```python
from build123d import *

# Parameters (mm, degrees)
CROQUIS1_W               = 28.88
CROQUIS1_H               = 55.3
CROQUIS1_R               = 1.5
SALIENTE_EXTRUIR8_DEPTH  = 3
CROQUIS19_W              = 28.88
CROQUIS19_H              = 55.3
CORTAR_EXTRUIR3_DEPTH    = 0.5
CROQUIS20_W              = 3
CROQUIS20_H              = 7.5
SALIENTE_EXTRUIR18_DEPTH = 23.5
SALIENTE_EXTRUIR19_START = -2.5
CROQUIS21_W              = 28.88
CROQUIS21_H              = 55.3
CROQUIS21_R              = 1.5
SALIENTE_EXTRUIR19_DEPTH = 2.5
CROQUIS22_R              = 1.5
CORTAR_EXTRUIR4_DEPTH    = 3
CROQUIS23_W              = 55.3
CROQUIS23_H              = 2.5
CORTAR_EXTRUIR5_DEPTH    = 68.588049239
CROQUIS24_W              = 55.3
CROQUIS24_H              = 23.5
SALIENTE_EXTRUIR20_DEPTH = 3


with BuildPart() as part:
    # Croquis1 → Saliente-Extruir8 (new body)
    with BuildSketch(Plane(origin=(0, 0, 0), x_dir=(1, 0, 0), z_dir=(0, 1, 0))):
        with Locations((14.44, 27.65)):
            Rectangle(CROQUIS1_W, CROQUIS1_H)
        with Locations(Location((14.44, 17.75, 0), (0, 0, 270))):
            Circle(CROQUIS1_R, mode=Mode.SUBTRACT)
        with Locations(Location((21.44, 17.75, 0), (0, 0, 270))):
            Circle(CROQUIS1_R, mode=Mode.SUBTRACT)
        with Locations(Location((14.44, 24.75, 0), (0, 0, 270))):
            Circle(CROQUIS1_R, mode=Mode.SUBTRACT)
        with Locations(Location((7.44, 17.75, 0), (0, 0, 270))):
            Circle(CROQUIS1_R, mode=Mode.SUBTRACT)
        with Locations(Location((14.44, 10.75, 0), (0, 0, 270))):
            Circle(CROQUIS1_R, mode=Mode.SUBTRACT)
        with Locations(Location((21.44, 37.55, 0), (0, 0, 90))):
            Circle(CROQUIS1_R, mode=Mode.SUBTRACT)
        with Locations(Location((14.44, 44.55, 0), (0, 0, 90))):
            Circle(CROQUIS1_R, mode=Mode.SUBTRACT)
        with Locations(Location((14.44, 30.55, 0), (0, 0, 90))):
            Circle(CROQUIS1_R, mode=Mode.SUBTRACT)
        with Locations(Location((14.44, 37.55, 0), (0, 0, 90))):
            Circle(CROQUIS1_R, mode=Mode.SUBTRACT)
        with Locations(Location((7.44, 37.55, 0), (0, 0, 90))):
            Circle(CROQUIS1_R, mode=Mode.SUBTRACT)
    extrude(amount=SALIENTE_EXTRUIR8_DEPTH)

    # Croquis19 → Cortar-Extruir3 (cut)
    with BuildSketch(Plane(origin=(0, 3, 0), x_dir=(1, 0, 0), z_dir=(0, 1, 0))):
        with Locations((14.44, 27.65)):
            Rectangle(CROQUIS19_W, CROQUIS19_H)
    extrude(amount=-CORTAR_EXTRUIR3_DEPTH, mode=Mode.SUBTRACT)

    # Croquis20 → Saliente-Extruir18 (add)
    with BuildSketch(Plane(origin=(0, 2.5, 0), x_dir=(1, 0, 0), z_dir=(0, 1, 0))):
        with Locations((1.5, 51.55)):
            Rectangle(CROQUIS20_W, CROQUIS20_H)
        with Locations((1.5, 3.75)):
            Rectangle(CROQUIS20_W, CROQUIS20_H)
    extrude(amount=SALIENTE_EXTRUIR18_DEPTH)

    # Croquis21 → Saliente-Extruir19 (add)
    with BuildSketch(Plane(origin=(0, 26, 0), x_dir=(1, 0, 0), z_dir=(0, 1, 0)).offset(SALIENTE_EXTRUIR19_START)):
        with Locations((14.44, 27.65)):
            Rectangle(CROQUIS21_W, CROQUIS21_H)
        with Locations(Location((14.44, 44.55, 0), (0, 0, 90))):
            Circle(CROQUIS21_R, mode=Mode.SUBTRACT)
        with Locations(Location((21.44, 37.55, 0), (0, 0, 90))):
            Circle(CROQUIS21_R, mode=Mode.SUBTRACT)
        with Locations(Location((14.44, 37.55, 0), (0, 0, 90))):
            Circle(CROQUIS21_R, mode=Mode.SUBTRACT)
        with Locations(Location((14.44, 30.55, 0), (0, 0, 90))):
            Circle(CROQUIS21_R, mode=Mode.SUBTRACT)
        with Locations(Location((7.44, 37.55, 0), (0, 0, 90))):
            Circle(CROQUIS21_R, mode=Mode.SUBTRACT)
        with Locations(Location((14.44, 24.75, 0), (0, 0, 270))):
            Circle(CROQUIS21_R, mode=Mode.SUBTRACT)
        with Locations(Location((21.44, 17.75, 0), (0, 0, 270))):
            Circle(CROQUIS21_R, mode=Mode.SUBTRACT)
        with Locations(Location((14.44, 17.75, 0), (0, 0, 270))):
            Circle(CROQUIS21_R, mode=Mode.SUBTRACT)
        with Locations(Location((7.44, 17.75, 0), (0, 0, 270))):
            Circle(CROQUIS21_R, mode=Mode.SUBTRACT)
        with Locations(Location((14.44, 10.75, 0), (0, 0, 270))):
            Circle(CROQUIS21_R, mode=Mode.SUBTRACT)
    extrude(amount=SALIENTE_EXTRUIR19_DEPTH)

    # Croquis22 → Cortar-Extruir4 (cut)
    with BuildSketch(Plane.ZY):
        with Locations((-51.3, 6.3)):
            Circle(CROQUIS22_R)
        with Locations((-51.3, 16.3)):
            Circle(CROQUIS22_R)
        with Locations(Location((-4, 16.3, 0), (0, 0, 180))):
            Circle(CROQUIS22_R)
        with Locations(Location((-4, 6.3, 0), (0, 0, 180))):
            Circle(CROQUIS22_R)
    extrude(amount=-CORTAR_EXTRUIR4_DEPTH, mode=Mode.SUBTRACT)

    # Croquis23 → Cortar-Extruir5 (cut, through all)
    with BuildSketch(Plane.ZY):
        with Locations((-27.65, 1.25)):
            Rectangle(CROQUIS23_W, CROQUIS23_H)
    extrude(amount=-CORTAR_EXTRUIR5_DEPTH, mode=Mode.SUBTRACT)

    # Croquis24 → Saliente-Extruir20 (add)
    with BuildSketch(Plane(origin=(28.88, 0, 0), x_dir=(0, 0, -1), z_dir=(1, 0, 0))):
        with Locations((27.65, 14.25)):
            Rectangle(CROQUIS24_W, CROQUIS24_H)
    extrude(amount=SALIENTE_EXTRUIR20_DEPTH)


solid = part.part
```
Verification items for the finished model (mm, model axes). A direction names the side the tool comes from. Give positions to 0.01 mm unless a question says otherwise; leave off trailing zeros. Order: outer loops, then holes, each group sorted by start corner. A loop starts at its lowest first (then second) coordinate and runs counter-clockwise, first axis right, second up. Notation, with made-up numbers: M 80.25,32 L 134.25,32 A19 cw 134.25,69 Z; hole C -30.5,-7.5 d8. An arc over 180 degrees is marked long. Answer in a Markdown table with one row per item. Add a question column.
Item 1: Tool access check on faces 1 (the flat face through (16, 26, -27)), 2 (the cylindrical face through (1.479, 14.836, -51.625)), 3 (the flat face through (1, 13, -7.5)). Record the directions out of +Z, -Z, +X, -X, +Y, -Y that give a thin tool (end or side, any length) a straight path to the whole face; none if there is none.
Item 2: Mould release check, pull along Z, two halves, no side actions. Record for faces 4 (the flat face through (15, 24, 0)), 5 (the cylindrical face through (14.51, 24.73, -19.25)), 6 (the flat face through (3, 13, -51)): released by +Z, released by -Z, zero draft, split by the parting line, or undercut.
Item 3: Section check B-B, the plane z = -24.75. Enter the section's corners in (x, y), and give its area (3 significant figures).
Item 4: Section check D-D, the plane z = -17.75. Enter the section's corners in (x, y), and give its area (3 significant figures).
Item 5: Section check C-C, the plane y = 11.5. Enter the section's corners in (x, z).
Item 6: Gauge pin test, flat end, axial feed: pin 1 (3.5 mm diameter, centred on x = 7.44, z = -37.55, fed in from -Y). Record the tip position at first contact, or that the pin passes through.
Item 7: Section check A-A, the plane x = 14.44. Enter the section's corners in (y, z), and give its area (4 significant figures).
Item 8: Scan lines: probe 1 along Y at (x, z) = (2.2, -4); probe 2 along X at (y, z) = (24.2, -30.55); probe 3 along X at (y, z) = (25.1, -17.75). Record each from-to range of solid material in increasing order. Write a range as from..to.
Filled sheet:
| question | item | result |
|---|---|---|
| 1 | face 1 | +Z, -Z, +X, -X, +Y |
| 1 | face 2 | -X |
| 1 | face 3 | -X, -Y |
| 2 | face 4 | released by +Z |
| 2 | face 5 | undercut |
| 2 | face 6 | zero draft |
| 3 | outline | M 0,23.5 L 12.94,23.5 L 12.94,26 L 0,26 Z; M 15.94,23.5 L 28.88,23.5 L 28.88,2.5 L 31.88,2.5 L 31.88,26 L 15.94,26 Z |
| 3 | area | 135 mm^2 |
| 4 | outline | M 0,23.5 L 5.94,23.5 L 5.94,26 L 0,26 Z; M 8.94,23.5 L 12.94,23.5 L 12.94,26 L 8.94,26 Z; M 15.94,23.5 L 19.94,23.5 L 19.94,26 L 15.94,26 Z; M 22.94,23.5 L 28.88,23.5 L 28.88,2.5 L 31.88,2.5 L 31.88,26 L 22.94,26 Z |
| 4 | area | 120 mm^2 |
| 5 | outline | M 0,-55.3 L 3,-55.3 L 3,-47.8 L 0,-47.8 Z; M 0,-7.5 L 3,-7.5 L 3,0 L 0,0 Z; M 28.88,-55.3 L 31.88,-55.3 L 31.88,0 L 28.88,0 Z |
| 6 | pin 1 | stops at y = 23.5 |
| 7 | outline | M 23.5,-55.3 L 26,-55.3 L 26,-46.05 L 23.5,-46.05 Z; M 23.5,-43.05 L 26,-43.05 L 26,-39.05 L 23.5,-39.05 Z; M 23.5,-36.05 L 26,-36.05 L 26,-32.05 L 23.5,-32.05 Z; M 23.5,-29.05 L 26,-29.05 L 26,-26.25 L 23.5,-26.25 Z; M 23.5,-23.25 L 26,-23.25 L 26,-19.25 L 23.5,-19.25 Z; M 23.5,-16.25 L 26,-16.25 L 26,-12.25 L 23.5,-12.25 Z; M 23.5,-9.25 L 26,-9.25 L 26,0 L 23.5,0 Z |
| 7 | area | 93.25 mm^2 |
| 8 | probe 1 | y = 2.5..4.8, 7.8..14.8, 17.8..26 |
| 8 | probe 2 | x = 0..12.94, 15.94..31.88 |
| 8 | probe 3 | x = 0..5.94, 8.94..12.94, 15.94..19.94, 22.94..31.88 |
